Design review of the part built by this model. Coordinates are the model's own, in mm. Face numbers are marked on the shaded views. A direction names the side the tool comes from. Coordinates: 2 decimals unless noted, no trailing zeros. Write each loop counter-clockwise with the first axis right and the second up, starting at its lowest first coordinate (ties: lowest second). Pieces come first, ordered by that corner, then holes. Notation, with made-up numbers: M 83,40 L 136,40 A22 cw 136,68 Z; hole C 20,56 d9. An arc over 180 degrees is marked long. Write item = value, one per line.
```python
from build123d import *

# Parameters (mm, degrees)
SKETCH1_R                             = 12.7
SKETCH1_R_2                           = 1.8288
BOSS_EXTRUDE1_DEPTH                   = 6.35
F_1_4_0_25_DIAMETER_HOLE1_D           = 6.35
F_1_4_0_25_DIAMETER_HOLE1_ON_FACE_2_D = 6.35
F_1_4_0_25_DIAMETER_HOLE1_ON_FACE_3_D = 6.35
F_1_4_0_25_DIAMETER_HOLE1_ON_FACE_4_D = 6.35
F_1_4_0_25_DIAMETER_HOLE1_ON_FACE_5_D = 6.35
F_1_4_0_25_DIAMETER_HOLE1_ON_FACE_6_D = 6.35
FILLET1_R                             = 3.175


with BuildPart() as part:
    # Sketch1 → Boss-Extrude1 (new, symmetric)
    with BuildSketch(Plane(origin=(0, 0, 0), x_dir=(1, 0, 0), z_dir=(0, 1, 0))):
        with BuildLine():
            Line((25.4, 4.7625), (25.4, -4.7625))
            Line((25.4, -4.7625), (50.8, -4.7625))
            Line((50.8, -4.7625), (50.8, -11.1125))
            Line((50.8, -11.1125), (22.84014763, -11.1125))
            ThreePointArc((22.84014763, -11.1125), (12.7, -21.997045256), (-1.796366515, -25.336398074))
            Line((-1.796366515, -25.336398074), (-15.7762927, -49.550340512))
            Line((-15.7762927, -49.550340512), (-21.275554014, -46.375340512))
            Line((-21.275554014, -46.375340512), (-8.575554014, -24.378295256))
            Line((-8.575554014, -24.378295256), (-16.824445986, -19.615795256))
            Line((-16.824445986, -19.615795256), (-29.524445986, -41.612840512))
            Line((-29.524445986, -41.612840512), (-35.0237073, -38.437840512))
            Line((-35.0237073, -38.437840512), (-21.043781114, -14.223898074))
            ThreePointArc((-21.043781114, -14.223898074), (-25.4, 0), (-21.043781114, 14.223898074))
            Line((-21.043781114, 14.223898074), (-35.0237073, 38.437840512))
            Line((-35.0237073, 38.437840512), (-29.524445986, 41.612840512))
            Line((-29.524445986, 41.612840512), (-16.824445986, 19.615795256))
            Line((-16.824445986, 19.615795256), (-8.575554014, 24.378295256))
            Line((-8.575554014, 24.378295256), (-21.275554014, 46.375340512))
            Line((-21.275554014, 46.375340512), (-15.7762927, 49.550340512))
            Line((-15.7762927, 49.550340512), (-1.796366515, 25.336398074))
            ThreePointArc((-1.796366515, 25.336398074), (12.7, 21.997045256), (22.84014763, 11.1125))
            Line((22.84014763, 11.1125), (50.8, 11.1125))
            Line((50.8, 11.1125), (50.8, 4.7625))
            Line((50.8, 4.7625), (25.4, 4.7625))
        make_face()
        with Locations(Location((0, 0, 0), (0, 0, 270))):
            Circle(SKETCH1_R, mode=Mode.SUBTRACT)
        with Locations(Location((-13.470384182, 13.470384182, 0), (0, 0, 270))):
            Circle(SKETCH1_R_2, mode=Mode.SUBTRACT)
        with Locations(Location((13.470384182, 13.470384182, 0), (0, 0, 270))):
            Circle(SKETCH1_R_2, mode=Mode.SUBTRACT)
        with Locations(Location((13.470384182, -13.470384182, 0), (0, 0, 270))):
            Circle(SKETCH1_R_2, mode=Mode.SUBTRACT)
        with Locations(Location((-13.470384182, -13.470384182, 0), (0, 0, 270))):
            Circle(SKETCH1_R_2, mode=Mode.SUBTRACT)
    extrude(amount=BOSS_EXTRUDE1_DEPTH, both=True)

    # 1/4 (0.25) Diameter Hole1 (through all)
    with Locations(Plane(origin=(38.1, 0, -4.7625), x_dir=(0, 1, 0), z_dir=(0, 0, 1))):
        with Locations((0, 0)):
            Hole(F_1_4_0_25_DIAMETER_HOLE1_D / 2)

    # 1/4 (0.25) Diameter Hole1 on face 2 (through all)
    with Locations(Plane(origin=(-14.925554014, 0, -35.376817884), x_dir=(-0.500000174844, 0, -0.866025302838), z_dir=(-0.866025302838, 0, 0.500000174844))):
        with Locations((0, 0)):
            Hole(F_1_4_0_25_DIAMETER_HOLE1_ON_FACE_2_D / 2)

    # 1/4 (0.25) Diameter Hole1 on face 3 (through all)
    with Locations(Plane(origin=(-23.174445986, 0, 30.614317884), x_dir=(-0.500000174844, 0, 0.866025302838), z_dir=(0.866025302838, 0, 0.500000174844))):
        with Locations((0, 0)):
            Hole(F_1_4_0_25_DIAMETER_HOLE1_ON_FACE_3_D / 2)

    # 1/4 (0.25) Diameter Hole1 on face 4 (through all)
    with Locations(Plane(origin=(-14.925554014, 0, 35.376817884), x_dir=(0.500000174844, 0, -0.866025302838), z_dir=(-0.866025302838, 0, -0.500000174844))):
        with Locations((0, 0)):
            Hole(F_1_4_0_25_DIAMETER_HOLE1_ON_FACE_4_D / 2)

    # 1/4 (0.25) Diameter Hole1 on face 5 (through all)
    with Locations(Plane(origin=(-23.174445986, 0, -30.614317884), x_dir=(0.500000174844, 0, 0.866025302838), z_dir=(0.866025302838, 0, -0.500000174844))):
        with Locations((0, 0)):
            Hole(F_1_4_0_25_DIAMETER_HOLE1_ON_FACE_5_D / 2)

    # 1/4 (0.25) Diameter Hole1 on face 6 (through all)
    with Locations(Plane(origin=(38.1, 0, 4.7625), x_dir=(-1, 0, 0), z_dir=(0, 0, -1))):
        with Locations((0, 0)):
            Hole(F_1_4_0_25_DIAMETER_HOLE1_ON_FACE_6_D / 2)

    # Fillet1
    fillet1_edges = [part.edges().sort_by_distance(p)[0] for p in [
        (25.4, 0, -4.7625),
        (22.84014763, 0, 11.1125),
        (-1.796366515, 0, 25.336398074),
        (-8.575554014, 0, 24.378295256),
        (-16.824445986, 0, 19.615795256),
        (-21.043781114, 0, 14.223898074),
        (-21.043781114, 0, -14.223898074),
        (-16.824445986, 0, -19.615795256),
        (-8.575554014, 0, -24.378295256),
        (-1.796366515, 0, -25.336398074),
        (22.84014763, 0, -11.1125),
    ]]
    fillet(fillet1_edges, radius=FILLET1_R)


solid = part.part
```
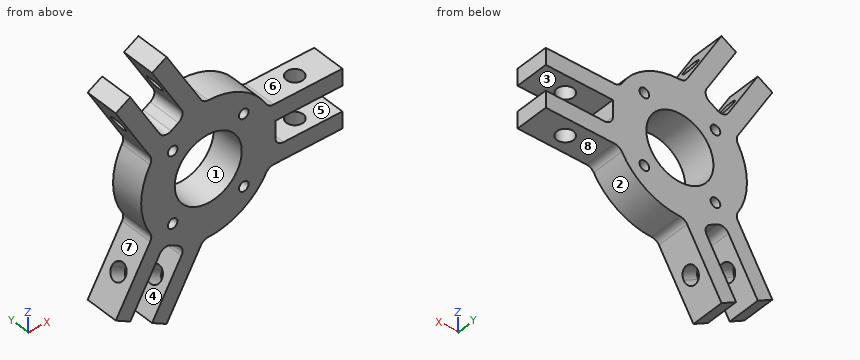
Q1. Consider section B-B, the plane z = 0. State the section outline as (x, y) points.
Check result:
outline = M -25.4,-6.35 L -12.7,-6.35 L -12.7,6.35 L -25.4,6.35 Z; M 12.7,-6.35 L 25.4,-6.35 L 25.4,6.35 L 12.7,6.35 Z
Q2. For P1, Ø6.5, axis at x = 34.5, y = 2.5, coming from the +Z side; P2, Ø1, axis at y = 0.5, z = 4.5, coming from the -X side; P3, Ø3, axis at y = -1, z = 0, coming from the +X side, all flat-tipped, find the tip position at first contact; note any pin that passes through.
Check result:
P1 = 11.11
P2 = -25.08
P3 = 25.4
Q3. Wall thickness on line 1 (X direction, y = 1.75, z = 0); line 2 (X direction, y = 2.5, z = 13); line 3 (Y direction, x = 38, z = 6): over which ranges is each line inside the solid? List them lowest first.
Check result:
line_1 = -25.4 to -12.7, 12.7 to 25.4
line_2 = -21.84 to -15.24, -11.7 to 11.7, 15.24 to 21.82
line_3 = -6.35 to -3.17, 3.17 to 6.35
Q4. Consider section A-A, the plane x = 42.5. State the section outline as (y, z) points.
Check result:
outline = M -6.35,-11.11 L 6.35,-11.11 L 6.35,-4.76 L -6.35,-4.76 Z; M -6.35,4.76 L 6.35,4.76 L 6.35,11.11 L -6.35,11.11 Z
Q5. Consider section C-C, the plane y = 0. State how many separate pieces and enclosed holes the cut face has, and give its area (3 significant figures).
Check result:
separate_pieces = 7
enclosed_holes = 5
area = 2,270 mm²
Q6. The part is to be moulded in two halves that separate along X. For the marked faces 1, 2 and 3, say which applies: +X half, -X half, draft (parallel to the pull), parting line (faces both ways), or undercut.
Check result:
face_1 = undercut
face_2 = +X half
face_3 = draft
Q7. Machinability: for the marked faces 4, 5, 6, 7 and 8, which of the approach directions +Z, -Z, +X, -X, +Y, -Y give a long, thin tool a straight path to every point of the face, cutting with its end or side? Answer none if there is none.
Check result:
face_4 = +Y, -Y
face_5 = +X, +Y, -Y
face_6 = +Z, +X, +Y, -Y
face_7 = -X, +Y, -Y
face_8 = -Z, +X, +Y, -Y
